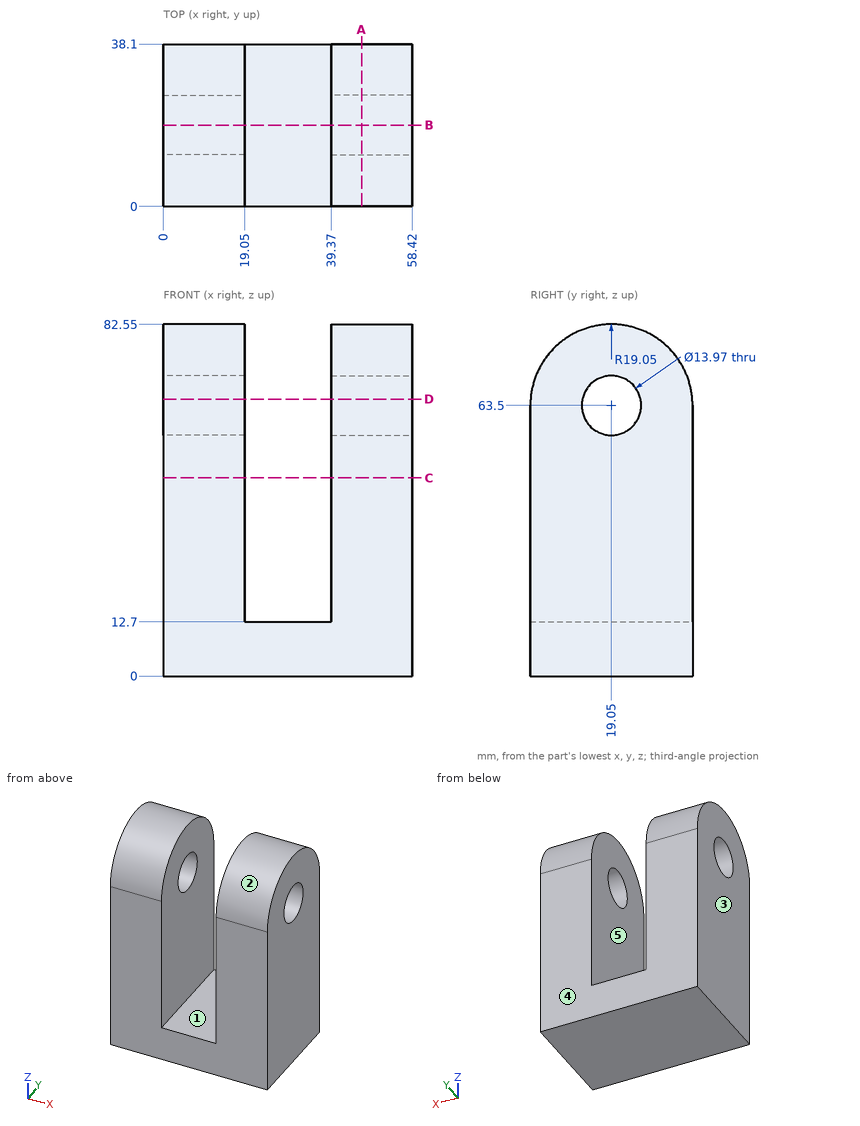
Source: three-view drawing plus pictorial views. Frame: mm from the lowest corner of the part. A direction names the side the tool comes from. Round coordinates to 2 decimals unless told otherwise and drop trailing zeros. Order: outer loops, then holes, each group sorted by start corner. A loop starts at its lowest first (then second) coordinate and runs counter-clockwise, first axis right, second up. Notation, with made-up numbers: (46.5, 29) - (77.5, 29) arc R28 cw to (77.5, 51) - close; hole circle Ø6 at (20, -23). An arc over 180 degrees is marked (long way). Answer in a Markdown table with one row per item.
Item 1: Mould query, pull axis X, two halves, no side actions, for the marked faces 1, 2 and 3. Classes: released by +X, released by -X, zero draft, split by the parting line, or undercut.
Model answer:
| item | result |
|---|---|
| face 1 | undercut |
| face 2 | zero draft |
| face 3 | released by -X |
Item 2: Section query C-C (z = 46.5). Return the cut outline in (x, y).
Model answer:
| item | result |
|---|---|
| outline | (0, 0) - (19.05, 0) - (19.05, 38.1) - (0, 38.1) - close; (39.37, 0) - (58.42, 0) - (58.42, 38.1) - (39.37, 38.1) - close |
Item 3: Section query A-A (x = 46.5). Return the cut outline in (y, z) (3 decimals), then the cut area to 3 significant figures.
Model answer:
| item | result |
|---|---|
| outline | (0, 0) - (38.1, 0) - (38.1, 63.5) arc R19.05 ccw to (0, 63.5) - close; hole circle Ø13.97 at (19.05, 63.5) |
| area | 2,840 mm² |
Item 4: Section query D-D (z = 65). Return the cut outline in (x, y).
Model answer:
| item | result |
|---|---|
| outline | (0, 0.06) - (19.05, 0.06) - (19.05, 12.23) - (0, 12.23) - close; (0, 25.87) - (19.05, 25.87) - (19.05, 38.04) - (0, 38.04) - close; (39.37, 0.06) - (58.42, 0.06) - (58.42, 12.23) - (39.37, 12.23) - close; (39.37, 25.87) - (58.42, 25.87) - (58.42, 38.04) - (39.37, 38.04) - close |
Item 5: Pin query (flat end, axial travel): pin 1 (8.5 mm diameter, centred on y = 19.05, z = 63.5, fed in from +X); pin 2 (16.5 mm diameter, centred on x = 30, y = 13.5, fed in from +Z). Return the tip coordinate at first contact, or that it passes through.
Model answer:
| item | result |
|---|---|
| pin 1 | passes through |
| pin 2 | stops at z = 12.7 |
Item 6: Line query: line 1 (X direction, y = 32, z = 45.5); line 2 (Z direction, x = 10, y = 19); line 3 (Y direction, x = 48, z = 63). Output: solid intervals per line, ascending.
Model answer:
| item | result |
|---|---|
| line 1 | x = 0 to 19.05, 39.37 to 58.42 |
| line 2 | z = 0 to 56.52, 70.48 to 82.55 |
| line 3 | y = 0 to 12.08, 26.02 to 38.1 |
Item 7: Reachability of the marked faces 4 and 5 from +Z, -Z, +X, -X, +Y, -Y: full face, straight path, thin tool, end or side. Return the list, or none.
Model answer:
| item | result |
|---|---|
| face 4 | +Z, -Z, +X, -X, +Y |
| face 5 | +Z, +Y, -Y |
Item 8: Section query B-B (y = 19.05). Return the cut outline in (x, z) (3 decimals), then the cut area to 3 significant figures.
Model answer:
| item | result |
|---|---|
| outline | (0, 0) - (58.42, 0) - (58.42, 56.515) - (39.37, 56.515) - (39.37, 12.7) - (19.05, 12.7) - (19.05, 56.515) - (0, 56.515) - close; (0, 70.485) - (19.05, 70.485) - (19.05, 82.55) - (0, 82.55) - close; (39.37, 70.485) - (58.42, 70.485) - (58.42, 82.55) - (39.37, 82.55) - close |
| area | 2,870 mm² |
